```python
from build123d import *

# Parameters (mm, degrees)
SKETCH1_W           = 1041.4
SKETCH1_H           = 304.8
BOSS_EXTRUDE1_DEPTH = 203.2
SKETCH3_R           = 57.15
BOSS_EXTRUDE2_DEPTH = 25.4
SKETCH4_R           = 57.15
BOSS_EXTRUDE3_DEPTH = 25.4
SKETCH5_W           = 990.6
SKETCH5_H           = 254
CUT_EXTRUDE1_DEPTH  = 177.8
SKETCH6_R           = 50.8
CUT_EXTRUDE2_DEPTH  = 177.8
SKETCH7_R           = 50.8
CUT_EXTRUDE3_DEPTH  = 177.8


with BuildPart() as part:
    # Sketch1 → Boss-Extrude1 (new body)
    with BuildSketch(Plane(origin=(0, 0, 0), x_dir=(1, 0, 0), z_dir=(0, 1, 0))):
        with Locations((520.7, 152.4)):
            Rectangle(SKETCH1_W, SKETCH1_H)
    extrude(amount=BOSS_EXTRUDE1_DEPTH)

    # Sketch3 → Boss-Extrude2 (add)
    with BuildSketch(Plane.XY):
        with Locations(Location((101.6, 101.6, 0), (0, 0, 180))):
            Circle(SKETCH3_R)
        with Locations(Location((381, 101.6, 0), (0, 0, 180))):
            Circle(SKETCH3_R)
        with Locations(Location((660.4, 101.6, 0), (0, 0, 180))):
            Circle(SKETCH3_R)
        with Locations(Location((939.8, 101.6, 0), (0, 0, 180))):
            Circle(SKETCH3_R)
    extrude(amount=BOSS_EXTRUDE2_DEPTH)

    # Sketch4 → Boss-Extrude3 (add)
    with BuildSketch(Plane(origin=(0, 0, -304.8), x_dir=(-1, 0, 0), z_dir=(0, 0, -1))):
        with Locations(Location((-508, 100.070914483, 0), (0, 0, 180))):
            Circle(SKETCH4_R)
    extrude(amount=BOSS_EXTRUDE3_DEPTH)

    # Sketch5 → Cut-Extrude1 (cut)
    with BuildSketch(Plane(origin=(0, 203.2, 0), x_dir=(1, 0, 0), z_dir=(0, 1, 0))):
        with Locations((520.7, 152.4)):
            Rectangle(SKETCH5_W, SKETCH5_H)
    extrude(amount=-CUT_EXTRUDE1_DEPTH, mode=Mode.SUBTRACT)

    # Sketch6 → Cut-Extrude2 (cut)
    with BuildSketch(Plane.XY.offset(25.4)):
        with Locations((101.6, 101.6)):
            Circle(SKETCH6_R)
        with Locations((381, 101.6)):
            Circle(SKETCH6_R)
        with Locations((660.4, 101.6)):
            Circle(SKETCH6_R)
        with Locations((939.8, 101.6)):
            Circle(SKETCH6_R)
    extrude(amount=-CUT_EXTRUDE2_DEPTH, mode=Mode.SUBTRACT)

    # Sketch7 → Cut-Extrude3 (cut)
    with BuildSketch(Plane(origin=(0, 0, -330.2), x_dir=(-1, 0, 0), z_dir=(0, 0, -1))):
        with Locations((-508, 100.070914483)):
            Circle(SKETCH7_R)
    extrude(amount=-CUT_EXTRUDE3_DEPTH, mode=Mode.SUBTRACT)


solid = part.part
```
Verification items for the finished model (mm, model axes). A direction names the side the tool comes from. Give positions to 0.01 mm unless a question says otherwise; leave off trailing zeros. Loops run counter-clockwise (first coordinate to the right, second up) from the corner with the lowest first, then second, coordinate; pieces in that order, holes last. Notation, with made-up numbers: M -29,80.25 L 16,80.25 A16 cw 16,97.25 Z; hole C -6,-24.5 d7. An arc over 180 degrees is marked long. Return JSON: item names as keys, results as strings.
1) Section check D-D, the plane x = 588.5. Enter the section's corners in (y, z), and give its area (3 significant figures).
Findings:
{"outline": "M 0,-304.8 L 203.2,-304.8 L 203.2,-279.4 L 25.4,-279.4 L 25.4,-25.4 L 203.2,-25.4 L 203.2,0 L 0,0 Z", "area": "16,800 mm2"}
2) Gauge pin test, flat ends, axial feed: P1, Ø5, axis at x = 359.5, y = 76, coming from the +Z side; P2, Ø12, axis at x = 232.5, y = 152, coming from the +Z side; P3, Ø4, axis at x = 119, y = 124, coming from the -Z side; P4, Ø10, axis at y = 77, z = -198, coming from the -X side. Record the tip position at first contact, or that the pin passes through.
Findings:
{"P1": "stops at z = -279.4", "P2": "stops at z = 0", "P3": "stops at z = -304.8", "P4": "stops at x = 0"}
3) Section check B-B, the plane z = -50. Enter the section's corners in (x, y), and give its area (3 significant figures).
Findings:
{"outline": "M 0,0 L 1041.4,0 L 1041.4,203.2 L 1016,203.2 L 1016,25.4 L 25.4,25.4 L 25.4,203.2 L 0,203.2 Z", "area": "35,500 mm2"}
4) Mould release check, pull along Y, two halves, no side actions. Record for faces 1 (the cylindrical face through (885.3, 84.4, 12.5)), 2 (the cylindrical face through (558.75, 102.3, -305.16)), 3 (the cylindrical face through (64.158, 135.933, 0.356)), 4 (the flat face through (140, 135.2, 25.4)): released by +Y, released by -Y, zero draft, split by the parting line, or undercut.
Findings:
{"face 1": "split by the parting line", "face 2": "undercut", "face 3": "undercut", "face 4": "zero draft"}
5) Material ranges on L1, parallel to X at y = 101, z = -13; L2, parallel to Z at x = 280.5, y = 177; L3, parallel to Y at x = 660, z = 7, recorded low to high. Write a range as [from, to].
Findings:
{"L1": "x = [0, 50.8], [152.4, 330.2], [431.8, 609.6], [711.2, 889], [990.6, 1041.4]", "L2": "z = [-304.8, -279.4], [-25.4, 0]", "L3": "y = [44.45, 50.8], [152.4, 158.75]"}
6) Section check C-C, the plane y = 170. Enter the section's corners in (x, z), and give its area (3 significant figures).
Findings:
{"outline": "M 0,-304.8 L 1041.4,-304.8 L 1041.4,0 L 0,0 Z; hole M 25.4,-279.4 L 1016,-279.4 L 1016,-25.4 L 25.4,-25.4 Z", "area": "65,800 mm2"}
7) Tool access check on faces 5 (the flat face through (419.4, 135.2, 25.4)), 6 (the cylindrical face through (560.79, 121.96, -317.32)), 7 (the flat face through (513, 100, 0)), 8 (the flat face through (514, 25.4, -154)). Record the directions out of +Z, -Z, +X, -X, +Y, -Y that give a thin tool (end or side, any length) a straight path to the whole face; none if there is none.
Findings:
{"face 5": "+Z, +X, -X, +Y, -Y", "face 6": "-Z", "face 7": "+Z", "face 8": "+Y"}
8) Section check A-A, the plane x = 939.8. Enter the section's corners in (y, z), and give its area (3 significant figures).
Findings:
{"outline": "M 0,-304.8 L 203.2,-304.8 L 203.2,-279.4 L 25.4,-279.4 L 25.4,-25.4 L 50.8,-25.4 L 50.8,25.4 L 44.45,25.4 L 44.45,0 L 0,0 Z; M 152.4,-25.4 L 203.2,-25.4 L 203.2,0 L 158.75,0 L 158.75,25.4 L 152.4,25.4 Z", "area": "14,500 mm2"}
